from build123d import *

# Parameters (mm, degrees)
SKETCH1_R           = 5
SKETCH1_R_2         = 1.75
BOSS_EXTRUDE1_DEPTH = 8.5
BOSS_EXTRUDE2_START = -8.5
BOSS_EXTRUDE2_DEPTH = 8.5


with BuildPart() as part:
    # Sketch1 → Boss-Extrude1 (new body)
    # profile 1 of 3: a face of its own
    with BuildSketch(Plane(origin=(0, 0, 0), x_dir=(1, 0, 0), z_dir=(0, 1, 0))):
        Circle(SKETCH1_R)
        with Locations(Location((0, 0, 0), (0, 0, 270))):
            Circle(SKETCH1_R_2, mode=Mode.SUBTRACT)
    # profile 2 of 3: a face of its own
    with BuildSketch(Plane(origin=(0, 0, 0), x_dir=(1, 0, 0), z_dir=(0, 1, 0))):
        with BuildLine():
            Line((22, 5), (0, 5))
            ThreePointArc((0, 5), (3.535533906, 3.535533906), (5, 0))
            ThreePointArc((5, 0), (3.535533907, -3.535533905), (3e-09, -5))
            Line((3e-09, -5), (22, -5))
            ThreePointArc((22, -5), (17, 0), (22, 5))
        make_face()
    # profile 3 of 3: a face of its own
    with BuildSketch(Plane(origin=(0, 0, 0), x_dir=(1, 0, 0), z_dir=(0, 1, 0))):
        with Locations((22, 0)):
            Circle(SKETCH1_R)
        with Locations(Location((22, 0, 0), (0, 0, 270))):
            Circle(SKETCH1_R_2, mode=Mode.SUBTRACT)
    extrude(amount=BOSS_EXTRUDE1_DEPTH)

    # Sketch2 → Boss-Extrude2 (add)
    with BuildSketch(Plane(origin=(0, 8.5, 0), x_dir=(1, 0, 0), z_dir=(0, 1, 0)).offset(BOSS_EXTRUDE2_START)):
        with BuildLine():
            ThreePointArc((22, 5), (27, 0), (22, -5))
            Line((22, -5), (24.99, -5))
            Line((24.99, -5), (31.08, -2.029708536))
            add(Edge.make_bspline(
                [(31.08, -2.029708536), (40.738723452, 6.188270814), (53.27, 6)],
                knots=[0, 0, 0, 1, 1, 1], degree=2))
            Line((53.27, 6), (60.557013712, 9.301428655))
            Line((60.557013712, 9.301428655), (58.75, 12.87))
            add(Edge.make_bspline(
                [(16.693950363, 5), (34.27932275, 6.303745675), (46.942612852, 18.996556194), (58.75, 12.87)],
                knots=[0.094833199, 0.094833199, 0.094833199, 0.094833199, 1, 1, 1, 1], degree=3))
            Line((16.693950363, 5), (22, 5))
        make_face()
    extrude(amount=BOSS_EXTRUDE2_DEPTH)


solid = part.part
For this review, take the finished solid that the model builds, in its own axes (mm). A direction names the side the tool comes from. Round coordinates to 2 decimals unless told otherwise and drop trailing zeros. Loops run counter-clockwise (first coordinate to the right, second up) from the corner with the lowest first, then second, coordinate; pieces in that order, holes last. Notation, with made-up numbers: (83.25, 9.25) - (121.25, 9.25) arc R14 ccw to (121.25, 34.25) - close; hole circle Ø4 at (71, -4). An arc over 180 degrees is marked (long way). One line per question, with ' | ' between items.
Q1. For pin 1 (1.5 mm diameter, centred on y = 7.5, z = -7, fed in from +X); pin 2 (1 mm diameter, centred on x = 53.5, y = 3, fed in from -Z), all flat-tipped, find the tip position at first contact; note any pin that passes through.
Taken from the geometry:
pin 1: stops at x = 57.13 | pin 2: stops at z = -14.49
Q2. Tool access review of faces 5 (the flat face through (56.862, 4.19, -7.628)), 6 (the flat face through (8, 4, -5)): name each direction out of +Z, -Z, +X, -X, +Y, -Y from which nothing blocks a thin tool from reaching the whole face with its end or side.
Taken from the geometry:
face 5: +Z, +X, +Y, -Y | face 6: -Z, -X, +Y, -Y
Q3. The part is to be moulded in two halves that separate along X. For faces 1 (the flat face through (59.666, 4.19, -11.061)), 2 (the cylindrical face through (-5, 4, 0)), 3 (the cylindrical face through (-1.71, 4.19, -0.38)), 4 (the flat face through (12, 4, 5)), say which applies: released by +X, released by -X, zero draft, split by the parting line, or undercut.
Taken from the geometry:
face 1: released by +X | face 2: released by -X | face 3: undercut | face 4: zero draft
Q4. Take a section at A-A (x = 14). Give the boundary of the cut face in (y, z), and give its area (3 significant figures).
Taken from the geometry:
outline: (0, -5) - (8.5, -5) - (8.5, 5) - (0, 5) - close | area: 85.0 mm²
Q5. Take a section at D-D (z = 3.5). Give the boundary of the cut face in (x, y).
Taken from the geometry:
outline: (-3.57, 0) - (28.07, 0) - (28.07, 8.5) - (-3.57, 8.5) - close
Q6. For line 1 along X through (y, z) = (3, 0); line 2 along X through (y, z) = (5.75, 1); line 3 along Z through (x, y) = (21.5, 7.25), list the stretches that pass through material, from the lowest coordinate up. Write a range as [from, to].
Taken from the geometry:
line 1: x = [-5, -1.75], [1.75, 20.25], [23.75, 33.69] | line 2: x = [-4.9, -1.44], [1.44, 20.56], [23.44, 32.34] | line 3: z = [-5.64, -1.68], [1.68, 5]
Q7. Take a section at B-B (z = 0). State how many separate pieces and enclosed holes the cut face has, and give its area (3 significant figures).
Taken from the geometry:
separate pieces: 3 | enclosed holes: 0 | area: 269 mm²
